The model under review builds one solid part; all positions refer to its coordinate system, in mm. Face numbers are marked on the shaded views. A direction names the side the tool comes from. Give positions to 0.01 mm unless a question says otherwise; leave off trailing zeros. Write each loop counter-clockwise with the first axis right and the second up, starting at its lowest first coordinate (ties: lowest second). Pieces come first, ordered by that corner, then holes.
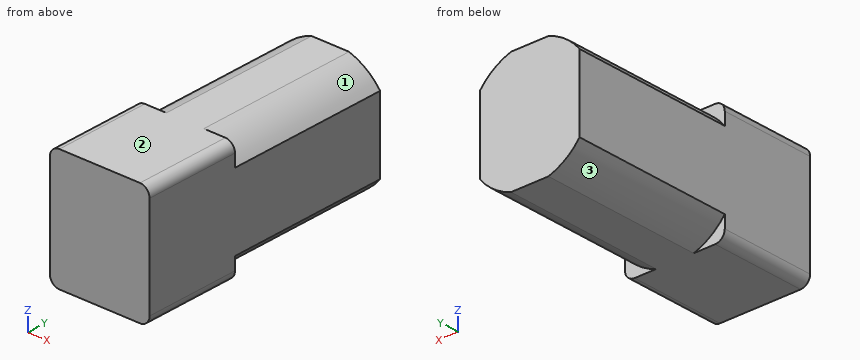
from build123d import *

# Parameters (mm, degrees)
BOX502_W                  = 10.4
BOX502_H                  = 12.4
BOX502_DEPTH              = 27
FILLET396_R               = 1
CYLINDER1193_R            = 8
CYLINDER1193_DEPTH        = 27
CYLINDER1195_R            = 6.5
CYLINDER1195_DEPTH        = 17
CYLINDER1194_R            = 8
CYLINDER1194_DEPTH        = 17
CYLINDER1196_R            = 8
CYLINDER1196_DEPTH        = 27
CUT014244_PLACEMENT_ANGLE = 90


with BuildPart() as fillet396:
    # Box502 → Box502 (new body)
    with BuildSketch(Plane(origin=(-5.2, -6.2, 0), x_dir=(1, 0, 0), z_dir=(0, 0, 1))):
        with Locations((5.2, 6.2)):
            Rectangle(BOX502_W, BOX502_H)
    extrude(amount=BOX502_DEPTH)

    # Fillet396
    fillet396_edges = [fillet396.edges().sort_by_distance(p)[0] for p in [
        (-5.2, -6.2, 13.5),
        (-5.2, 6.2, 13.5),
        (5.2, -6.2, 13.5),
        (5.2, 6.2, 13.5),
    ]]
    fillet(fillet396_edges, radius=FILLET396_R)


with BuildPart() as cut014243:
    # Cylinder1193 → Cylinder1193 (new body)
    with BuildSketch(Plane.XY):
        Circle(CYLINDER1193_R)
    extrude(amount=CYLINDER1193_DEPTH)

    # Cut014243: cut Fillet396
    add(fillet396.part, mode=Mode.SUBTRACT)


with BuildPart() as cylinder1413:
    # Cylinder1195 → Cylinder1195 (new body)
    with BuildSketch(Plane.XY):
        Circle(CYLINDER1195_R)
    extrude(amount=CYLINDER1195_DEPTH)


with BuildPart() as fusion248002050122:
    # Cylinder1194 → Cylinder1194 (new body)
    with BuildSketch(Plane.XY):
        Circle(CYLINDER1194_R)
    extrude(amount=CYLINDER1194_DEPTH)

    # Cut014242: cut Cylinder1413
    add(cylinder1413.part, mode=Mode.SUBTRACT)

    # Fusion248002050122: union Cut014243
    add(cut014243.part)


with BuildPart() as bucket_turning_motor:
    # Cylinder1196 → Cylinder1196 (new body)
    with BuildSketch(Plane.XY):
        Circle(CYLINDER1196_R)
    extrude(amount=CYLINDER1196_DEPTH)

    # Cut014244: cut Fusion248002050122
    add(fusion248002050122.part, mode=Mode.SUBTRACT)


with BuildPart() as bucket_turning_motor_1:
    # Cut014244 placement: moved
    add(bucket_turning_motor.part.moved(Location((480.5, 119, 114.75))).rotate(Axis((480.5, 119, 114.75), (1, 0, 0)), CUT014244_PLACEMENT_ANGLE))


solid = bucket_turning_motor_1.part
1) To check wall thickness, follow probe 1 along Z at (x, y) = (482.5, 115.25); probe 2 along Z at (x, y) = (476, 115.25); probe 3 along X at (y, z) = (102.5, 120.25). State the ranges of each line that lie inside material, in increasing order.
2) Insertion check: pin 1 (1.8 mm diameter, centred on x = 484.5, z = 120, fed in from +Y); pin 2 (1.5 mm diameter, centred on x = 477, y = 112.5, fed in from -Z). Each pin has a flat end and moves straight along its axis. Give the tip position at first contact, or say it passes through.
3) Tool access review of the marked faces 1, 2 and 3: name each direction out of +Z, -Z, +X, -X, +Y, -Y from which nothing blocks a thin tool from reaching the whole face with its end or side.
4) Consider section A-A, the plane y = 111. Give the boundary of the cut face in (x, z), then the cut area to 3 significant figures.
5) Consider section B-B, the plane z = 110.5. Give the boundary of the cut face in (x, y).
Answer block:
1. probe 1: z = 108.57 to 120.93
1. probe 2: z = 110.06 to 119.44
1. probe 3: x = 477.04 to 483.96
2. pin 1: stops at y = 119
2. pin 2: stops at z = 108.86
3. face 1: +Z, +X, +Y
3. face 2: +Z, +X, -X, +Y, -Y
3. face 3: -Z, -X, +Y
4. outline: (475.3, 110.85) arc R6.5 ccw to (478.55, 108.55) - (482.45, 108.55) arc R6.5 ccw to (485.7, 110.85) - (485.7, 118.65) arc R6.5 ccw to (482.45, 120.95) - (478.55, 120.95) arc R6.5 ccw to (475.3, 118.65) - close
4. area: 117 mm2
5. outline: (475.3, 92) - (485.7, 92) - (485.7, 102) - (485.42, 102) - (485.42, 119) - (475.58, 119) - (475.58, 102) - (475.3, 102) - close
